Input: dimensioned drawing with shaded views. Units: mm. Origin: part minimum x, y, z. A direction names the side the tool comes from. Round coordinates to 2 decimals unless told otherwise and drop trailing zeros. Loops run counter-clockwise (first coordinate to the right, second up) from the corner with the lowest first, then second, coordinate; pieces in that order, holes last. Notation, with made-up numbers: (87, 23) - (95, 23) arc R26 ccw to (95, 60) - close; hole circle Ø5 at (-36, 50.5). An arc over 180 degrees is marked (long way). Use CSV: the item, a comma, the result in double quotes. Start each with the question number.
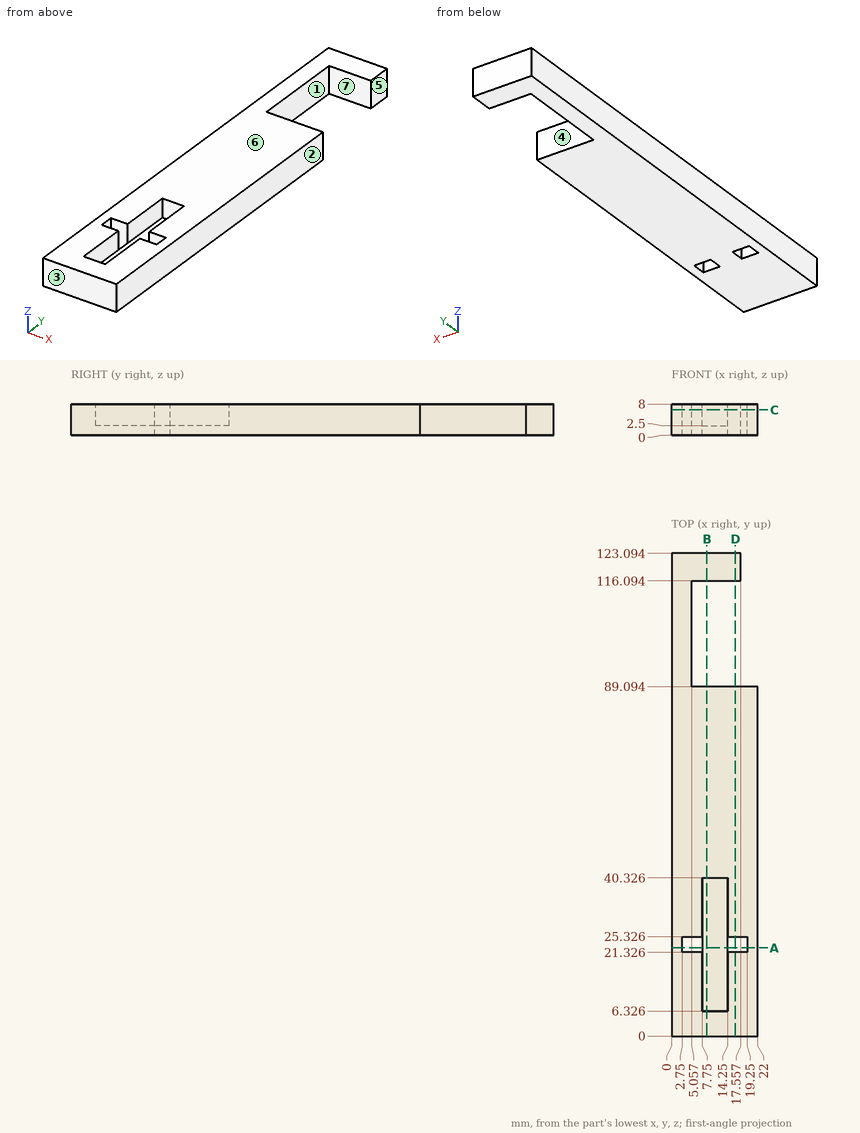
1. Section query A-A on y = 22.5. Return the cut outline in (x, z).
2. Contact query for flat-ended pins moving along their axis: P1, Ø2, axis at y = 120, z = 3.5, coming from the +X side; P2, Ø2, axis at y = 95.5, z = 5, coming from the +X side. Output: stop coordinate, or through.
3. Mould query, pull axis Y, two halves, no side actions, for the marked faces 1, 2, 3 and 4. Classes: +Y half, -Y half, draft (parallel to the pull), parting line (faces both ways), or undercut.
4. Line query: line 1 along Y through (x, z) = (6, 2.5); line 2 along X through (y, z) = (36, 5.75); line 3 along Y through (x, z) = (3.75, 4). Output: solid intervals per line, ascending.
5. Reachability of the marked faces 5, 6 and 7 from +Z, -Z, +X, -X, +Y, -Y: full face, straight path, thin tool, end or side. Return the list, or none.
6. Section query D-D on x = 16.25. Return the cut outline in (y, z), and give its area (3 significant figures).
7. Section query B-B on x = 9. Return the cut outline in (y, z), and give its area (3 significant figures).
8. Section query C-C on z = 6.5. Return the cut outline in (x, y), and give its area (3 significant figures).
Values:
1,outline,"(0, 0) - (2.75, 0) - (2.75, 8) - (0, 8) - close; (7.75, 0) - (14.25, 0) - (14.25, 2.5) - (7.75, 2.5) - close; (19.25, 0) - (22, 0) - (22, 8) - (19.25, 8) - close"
2,P1,"stops at x = 17.56"
2,P2,"stops at x = 5.06"
3,face 1,"undercut"
3,face 2,"draft"
3,face 3,"-Y half"
3,face 4,"undercut"
4,line 1,"y = 0 to 21.33, 25.33 to 89.09, 116.09 to 123.09"
4,line 2,"x = 0 to 7.75, 14.25 to 22"
4,line 3,"y = 0 to 21.33, 25.33 to 123.09"
5,face 5,"+Z, -Z, +X, +Y"
5,face 6,"+Z, +X, -X, +Y, -Y"
5,face 7,"+Z, -Z, +X"
6,outline,"(0, 0) - (21.33, 0) - (21.33, 8) - (0, 8) - close; (25.33, 0) - (89.09, 0) - (89.09, 8) - (25.33, 8) - close; (116.09, 0) - (123.09, 0) - (123.09, 8) - (116.09, 8) - close"
6,area,"737 mm^2"
7,outline,"(0, 0) - (89.09, 0) - (89.09, 8) - (40.33, 8) - (40.33, 2.5) - (6.33, 2.5) - (6.33, 8) - (0, 8) - close; (116.09, 0) - (123.09, 0) - (123.09, 8) - (116.09, 8) - close"
7,area,"582 mm^2"
8,outline,"(0, 0) - (22, 0) - (22, 89.09) - (5.06, 89.09) - (5.06, 116.09) - (17.56, 116.09) - (17.56, 123.09) - (0, 123.09) - close; hole (2.75, 21.33) - (7.75, 21.33) - (7.75, 6.33) - (14.25, 6.33) - (14.25, 21.33) - (19.25, 21.33) - (19.25, 25.33) - (14.25, 25.33) - (14.25, 40.33) - (7.75, 40.33) - (7.75, 25.33) - (2.75, 25.33) - close"
8,area,"1,960 mm^2"
